from build123d import *

# Parameters (mm, degrees)
SKETCH1_W           = 300
SKETCH1_H           = 260
BOSS_EXTRUDE1_DEPTH = 10
SKETCH2_R           = 10
CUT_EXTRUDE1_DEPTH  = 199.746069144
LPATTERN1_COUNT     = 4
LPATTERN1_PITCH     = 60


with BuildPart() as part:
    # Sketch1 → Boss-Extrude1 (new body)
    with BuildSketch(Plane(origin=(0, 0, 0), x_dir=(1, 0, 0), z_dir=(0, 1, 0))):
        Rectangle(SKETCH1_W, SKETCH1_H)
    extrude(amount=BOSS_EXTRUDE1_DEPTH)

    # Sketch2 → Cut-Extrude1 (cut, through all)
    with BuildSketch(Plane(origin=(0, 10, 0), x_dir=(1, 0, 0), z_dir=(0, 1, 0))):
        with Locations(Location((-90, -100, 0), (0, 0, 270))):
            Circle(SKETCH2_R)
    cut_extrude1 = extrude(amount=-CUT_EXTRUDE1_DEPTH, mode=Mode.SUBTRACT)

    # LPattern1: Cut-Extrude1 ×4
    with Locations(*[(i * LPATTERN1_PITCH, 0, 0) for i in range(1, LPATTERN1_COUNT)]):
        add(cut_extrude1, mode=Mode.SUBTRACT)


solid = part.part
Geometry: final body of the model. Coordinates: model frame, mm. Give positions to 0.01 mm unless a question says otherwise; leave off trailing zeros. Write each loop counter-clockwise with the first axis right and the second up, starting at its lowest first coordinate (ties: lowest second). Pieces come first, ordered by that corner, then holes. Notation, with made-up numbers: (56, -20) - (66, -20) arc R26 ccw to (66, 10) - close; hole circle Ø1 at (74.25, 84.5). An arc over 180 degrees is marked (long way). Return JSON: item names as keys, results as strings. Group by question number.
1) Line query: line 1 (X direction, y = 2.5, z = 100); line 2 (X direction, y = 9.25, z = 98). Output: solid intervals per line, ascending.
2) First-contact query: P1, Ø5, axis at x = -74.5, z = 67.5, coming from the -Y side; P2, Ø16, axis at x = -90, z = 100, coming from the +Y side. Flat tips, straight axial feed; report the tip coordinate or a pass-through.
3) Section C-C on z = 100. Return the cut outline in (x, y), plus the area to 3 significant figures.
4) Section B-B on x = -90. Return the cut outline in (y, z), plus the area to 3 significant figures.
5) Section A-A on y = 3. Return the cut outline in (x, z), plus the area to 3 significant figures.
6) Mould query, pull axis Z, two halves, no side actions, for faces 1 (the cylindrical face through (-80.085, 5.07, 98.698)), 2 (the cylindrical face through (-36, 5, 92)), 3 (the flat face through (-2, 10, -2)), 4 (the flat face through (-2, 5, 130)). Classes: released by +Z, released by -Z, zero draft, split by the parting line, or undercut.
Filled in:
{
 "1": {"line 1": "x = -150 to -100, -80 to -40, -20 to 20, 40 to 80, 100 to 150", "line 2": "x = -150 to -99.8, -80.2 to -39.8, -20.2 to 20.2, 39.8 to 80.2, 99.8 to 150"},
 "2": {"P1": "stops at y = 0", "P2": "passes through"},
 "3": {"outline": "(-150, 0) - (-100, 0) - (-100, 10) - (-150, 10) - close; (-80, 0) - (-40, 0) - (-40, 10) - (-80, 10) - close; (-20, 0) - (20, 0) - (20, 10) - (-20, 10) - close; (40, 0) - (80, 0) - (80, 10) - (40, 10) - close; (100, 0) - (150, 0) - (150, 10) - (100, 10) - close", "area": "2,200 mm^2"},
 "4": {"outline": "(0, -130) - (10, -130) - (10, 90) - (0, 90) - close; (0, 110) - (10, 110) - (10, 130) - (0, 130) - close", "area": "2,400 mm^2"},
 "5": {"outline": "(-150, -130) - (150, -130) - (150, 130) - (-150, 130) - close; hole circle Ø20 at (-90, 100); hole circle Ø20 at (-30, 100); hole circle Ø20 at (30, 100); hole circle Ø20 at (90, 100)", "area": "76,700 mm^2"},
 "6": {"face 1": "undercut", "face 2": "undercut", "face 3": "zero draft", "face 4": "released by +Z"}
}
